Read the model definition and answer for the solid it produces. Units are mm, in the model's axes. A direction names the side the tool comes from. Round coordinates to 2 decimals unless told otherwise and drop trailing zeros. Loops run counter-clockwise (first coordinate to the right, second up) from the corner with the lowest first, then second, coordinate; pieces in that order, holes last. Notation, with made-up numbers: (-9, 8) - (44, 8) arc R8 cw to (44, 20) - close; hole circle Ø11 at (46.25, -24.75). An arc over 180 degrees is marked (long way). Use CSV: the item, a comma, the result in double quotes. Start each with the question number.
1. Find section A-A (x = 14.9). Give the vertices of the cut face in (y, z), and give its area (3 significant figures).
2. Find section C-C (z = 17). Give the vertices of the cut face in (x, y), and give its area (4 significant figures).
3. A tool of negligible diameter and unlimited length cuts with its end or side. For faces 5 (the flat face through (8.5, 4, 17)), 6 (the flat face through (43, 6, 28)), 7 (the flat face through (3, 7, 11)), 8 (the cylindrical face through (-4.437, 12.266, 5.479)), from which of +Z, -Z, +X, -X, +Y, -Y can it reach the whole face along a straight path? Write none if from no direction.
4. Given pin 1 Ø5 at (x, z) = (35.5, 18.5) entering from +Y; pin 2 Ø3 at (y, z) = (7, 16.5) entering from -X; pin 3 Ø5.5 at (x, y) = (3.5, 5) entering from -Z; pin 4 Ø2.5 at (x, z) = (14.9, 30.9) entering from -Y (3 decimals), each flat-ended and moving along its own axis, determine where each tip first touches the part or whether it passes through.
5. Find section B-B (y = 8.3). Give the vertices of the cut face in (x, z), and give its area (3 significant figures).
6. Determine the mould class of faces 1 (the flat face through (43, 6, 1)), 2 (the flat face through (3, 7, 33)), 3 (the flat face through (-9, 8, 28)), 4 (the flat face through (3, 7, 23)) for opening direction Z: +Z half, -Z half, draft (parallel to the pull), parting line (faces both ways), or undercut.
7. Consider line 1 along X through (y, z) = (0.4, 3.1); line 2 along Z through (x, y) = (14.9, 1.15); line 3 along X through (y, z) = (10, 4). Determine where each line is inside the solid, lowest interval first.
8. Find section D-D (z = 6). Give the vertices of the cut face in (x, y), and give its area (4 significant figures).
from build123d import *

# Parameters (mm, degrees)
SKETCH1_W           = 55
SKETCH1_H           = 34
BOSS_EXTRUDE1_DEPTH = 1.5
SKETCH2_R           = 1.9
CUT_EXTRUDE1_DEPTH  = 2.5
FILLET1_R           = 3
SKETCH3_W           = 8
SKETCH3_H           = 5
BOSS_EXTRUDE2_DEPTH = 5
SKETCH4_R           = 2.25
BOSS_EXTRUDE3_DEPTH = 2
SKETCH5_W           = 3
SKETCH5_H           = 27
BOSS_EXTRUDE4_DEPTH = 10
SKETCH6_W           = 6
SKETCH6_H           = 10
BOSS_EXTRUDE5_DEPTH = 11
SKETCH7_R           = 4
BOSS_EXTRUDE6_DEPTH = 9


with BuildPart() as part:
    # Sketch1 → Boss-Extrude1 (new body)
    with BuildSketch(Plane(origin=(0, 0, 0), x_dir=(1, 0, 0), z_dir=(0, 1, 0))):
        with Locations((27.5, -17)):
            Rectangle(SKETCH1_W, SKETCH1_H)
    extrude(amount=BOSS_EXTRUDE1_DEPTH)

    # Sketch2 → Cut-Extrude1 (cut, through all)
    with BuildSketch(Plane(origin=(0, 1.5, 0), x_dir=(1, 0, 0), z_dir=(0, 1, 0))):
        with Locations((51.9, -30.9)):
            Circle(SKETCH2_R)
        with Locations((14.9, -30.9)):
            Circle(SKETCH2_R)
        with Locations((14.9, -3.1)):
            Circle(SKETCH2_R)
        with Locations((51.9, -3.1)):
            Circle(SKETCH2_R)
    extrude(amount=-CUT_EXTRUDE1_DEPTH, mode=Mode.SUBTRACT)

    # Fillet1
    fillet1_edges = [part.edges().sort_by_distance(p)[0] for p in [
        (55, 0.75, 0),
        (55, 0.75, 34),
    ]]
    fillet(fillet1_edges, radius=FILLET1_R)

    # Sketch3 → Boss-Extrude2 (add)
    with BuildSketch(Plane(origin=(0, 1.5, 0), x_dir=(1, 0, 0), z_dir=(0, 1, 0))):
        with Locations((4.5, -17)):
            Rectangle(SKETCH3_W, SKETCH3_H)
    extrude(amount=BOSS_EXTRUDE2_DEPTH)

    # Sketch4 → Boss-Extrude3 (add)
    with BuildSketch(Plane.ZY.offset(-0.5)):
        with Locations((17, 4)):
            Circle(SKETCH4_R)
    extrude(amount=BOSS_EXTRUDE3_DEPTH)

    # Sketch5 → Boss-Extrude4 (add)
    with BuildSketch(Plane(origin=(0, 1.5, 0), x_dir=(1, 0, 0), z_dir=(0, 1, 0))):
        with Locations((43.5, -14.5)):
            Rectangle(SKETCH5_W, SKETCH5_H)
    extrude(amount=BOSS_EXTRUDE4_DEPTH)

    # Sketch6 → Boss-Extrude5 (add)
    with BuildSketch(Plane(origin=(0, 1.5, 0), x_dir=(1, 0, 0), z_dir=(0, 1, 0))):
        with Locations((3, -6)):
            Rectangle(SKETCH6_W, SKETCH6_H)
        with Locations((3, -28)):
            Rectangle(SKETCH6_W, SKETCH6_H)
    extrude(amount=BOSS_EXTRUDE5_DEPTH)

    # Sketch7 → Boss-Extrude6 (add)
    with BuildSketch(Plane.ZY):
        with Locations((28, 8.3)):
            Circle(SKETCH7_R)
        with Locations((6, 8.3)):
            Circle(SKETCH7_R)
    extrude(amount=BOSS_EXTRUDE6_DEPTH)


solid = part.part
Filled sheet:
1,outline,"(0, 0) - (1.5, 0) - (1.5, 1.2) - (0, 1.2) - close; (0, 5) - (1.5, 5) - (1.5, 29) - (0, 29) - close; (0, 32.8) - (1.5, 32.8) - (1.5, 34) - (0, 34) - close"
1,area,"39.6 mm²"
2,outline,"(-1.5, 1.75) - (0.5, 1.75) - (0.5, 1.5) - (0, 1.5) - (0, 0) - (55, 0) - (55, 1.5) - (45, 1.5) - (45, 11.5) - (42, 11.5) - (42, 1.5) - (8.5, 1.5) - (8.5, 6.5) - (0.5, 6.5) - (0.5, 6.25) - (-1.5, 6.25) - close"
2,area,"161.5 mm²"
3,face 5,"+Z, -Z, +Y"
3,face 6,"+Z, +X, +Y"
3,face 7,"-X, +Y"
3,face 8,"-X"
4,pin 1,"stops at y = 1.5"
4,pin 2,"stops at x = -1.5"
4,pin 3,"stops at z = 1"
4,pin 4,"passes through"
5,outline,"(-9, 2) - (0, 2) - (0, 1) - (6, 1) - (6, 11) - (0, 11) - (0, 10) - (-9, 10) - close; (-9, 24) - (0, 24) - (0, 23) - (6, 23) - (6, 33) - (0, 33) - (0, 32) - (-9, 32) - close; (42, 1) - (45, 1) - (45, 28) - (42, 28) - close"
5,area,"345 mm²"
6,face 1,"-Z half"
6,face 2,"+Z half"
6,face 3,"draft"
6,face 4,"undercut"
7,line 1,"x = 0 to 13, 16.8 to 50, 53.8 to 55"
7,line 2,"z = 0 to 1.2, 5 to 29, 32.8 to 34"
7,line 3,"x = -9 to 6, 42 to 45"
8,outline,"(-9, 4.3) - (0, 4.3) - (0, 0) - (55, 0) - (55, 1.5) - (45, 1.5) - (45, 11.5) - (42, 11.5) - (42, 1.5) - (6, 1.5) - (6, 12.5) - (0, 12.5) - (0, 12.3) - (-9, 12.3) - close"
8,area,"250.5 mm²"
